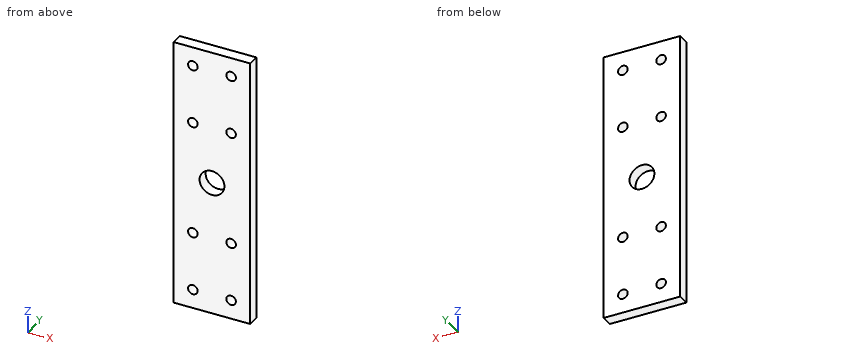
Autodesk Inventor part; units mm, degrees
ref_plane "YZ Plane" through (0, 0, 0) normal (1, 0, 0) x (0, 1, 0)
ref_plane "XZ Plane" through (0, 0, 0) normal (0, 1, 0) x (-1, 0, 0)
ref_plane "XY Plane" through (0, 0, 0) normal (0, 0, 1) x (1, 0, 0)
sketch "Esboço1" plane through (0, 0, 0) normal (0, 1, 0) x (-1, 0, 0)
  line L0 (0, 0) -> (40, 0)
  line L1 (40, 0) -> (40, -142)
  line L2 (40, -142) -> (0, -142)
  line L3 (0, -142) -> (0, 0)
  dimension "d0" = 40
  dimension "d1" = 142
extrude "Extrusão1" add sketch "Esboço1" along normal blind 6
sketch "Esboço2" plane through (0, 6, 0) normal (0, 1, 0) x (1, 0, 0)
  line L0 (-40, 142) -> (-40, 0)
  line L1 (-40, 0) -> (0, 0)
  point P0 (-20, 71)
  dimension "d4" = 142
  dimension "d5" = 40
  dimension "d6" = 20
  dimension "d7" = 71
hole "Furo1" at (-20, 6, -71) direction (0, -1, 0) diameter 13 depth 6
sketch "Esboço4" plane through (0, 6, 0) normal (0, 1, 0) x (1, 0, 0)
  line L0 (0, 142) -> (-40, 142)
  line L1 (0, 0) -> (0, 142)
  line L2 (-40, 0) -> (0, 0)
  line L3 (-40, 142) -> (-40, 0)
  circle A0 centre (-20, 71) radius 6.5
  point P0 (-10, 10)
  point P1 (-10, 132)
  point P2 (-20, 0)
  point P3 (-30, 132)
  point P4 (-30, 10)
  point P5 (-30, 101)
  point P6 (-10, 101)
  point P7 (-10, 41)
  point P8 (-30, 41)
  dimension "d45" = 40
  dimension "d46" = 10
  dimension "d47" = 10
  dimension "d48" = 10
  dimension "d49" = 10
  dimension "d57" = 10
  dimension "d58" = 10
  dimension "d59" = 10
  dimension "d60" = 60
  dimension "d61" = 30
hole "Furo3" at (-10, 6, -10) at (-10, 6, -132) at (-30, 6, -10) at (-30, 6, -132) at (-30, 6, -41) at (-10, 6, -41) at (-30, 6, -101) at (-10, 6, -101) direction (0, -1, 0) diameter 5 end through all
equation "\"d13\" = Espessura"
equation "\"d55\" = Espessura"
equation "\"Raio_vergadura\" = Espessura"
equation "\"Largura_alívio_de_vergadura\" = Espessura"
equation "\"Profundidade_alívio_de_vergadura\" = 0.5 * Espessura"
equation "\"Tamanho_alívio_de_dobra\" = 4 * Espessura"
equation "\"Remanescente_mínimo\" = 2 * Espessura"
equation "\"Raiodetransição\" = Raio_vergadura"
equation "\"Tamanho_de_raio_de_Jacobi\" = Raio_vergadura"
equation "\"TamanhoFolga\" = Espessura"
properties part number "Suporte superior do eixo" material "Aluminum 6061"
Part model, mm, in its own coordinate system. Coordinates: 2 decimals unless noted, no trailing zeros. Order: outer loops, then holes, each group sorted by start corner. A loop starts at its lowest first (then second) coordinate and runs counter-clockwise, first axis right, second up. Notation, with made-up numbers: M -25.5,73.5 L 2.5,73.5 A9 ccw 2.5,85.5 Z; hole C 29,12 d2. An arc over 180 degrees is marked long. Use a Markdown table: item, result.
(1) Cut at C-C on z = -10. Write the cut outline in (x, y), then the cut area to 3 significant figures.
A:
| item | result |
|---|---|
| outline | M -40,0 L -32.5,0 L -32.5,6 L -40,6 Z; M -27.5,0 L -12.5,0 L -12.5,6 L -27.5,6 Z; M -7.5,0 L 0,0 L 0,6 L -7.5,6 Z |
| area | 180 mm^2 |
(2) Cut at B-B on z = -71. Write the cut outline in (x, y), then the cut area to 3 significant figures.
A:
| item | result |
|---|---|
| outline | M -40,0 L -26.5,0 L -26.5,6 L -40,6 Z; M -13.5,0 L 0,0 L 0,6 L -13.5,6 Z |
| area | 162 mm^2 |
(3) Probe L1, parallel to Z at x = -10, y = 2.35; L2, parallel to X at y = 4.1, z = -101; L3, parallel to Z at x = -32, y = 3.75. List the from-to ranges inside material, lowest first.
A:
| item | result |
|---|---|
| L1 | z = -142 to -134.5, -129.5 to -103.5, -98.5 to -43.5, -38.5 to -12.5, -7.5 to 0 |
| L2 | x = -40 to -32.5, -27.5 to -12.5, -7.5 to 0 |
| L3 | z = -142 to -133.5, -130.5 to -102.5, -99.5 to -42.5, -39.5 to -11.5, -8.5 to 0 |
(4) Cut at D-D on y = 2.35. State how many separate pieces and enclosed holes the cut face has, then the cut area to 3 significant figures.
A:
| item | result |
|---|---|
| separate pieces | 1 |
| enclosed holes | 9 |
| area | 5,390 mm^2 |
(5) Cut at A-A on x = -20. Write the cut outline in (y, z), then the cut area to 3 significant figures.
A:
| item | result |
|---|---|
| outline | M 0,-142 L 6,-142 L 6,-77.5 L 0,-77.5 Z; M 0,-64.5 L 6,-64.5 L 6,0 L 0,0 Z |
| area | 774 mm^2 |
